Can you work these out from the drawing? Everything is in mm from the part's minimum corner. A direction names the side the tool comes from. Round coordinates to 2 decimals unless told otherwise and drop trailing zeros. Loops run counter-clockwise (first coordinate to the right, second up) from the corner with the lowest first, then second, coordinate; pieces in that order, holes last. Notation, with made-up numbers: (56.5, 6) - (108.5, 6) arc R5 ccw to (108.5, 10) - close; hole circle Ø11 at (55.25, -19). An arc over 180 degrees is marked (long way). Answer as a JSON object with one key per item and string values. Group by question number.
1) I want a section at B-B, the plane x = 30.5. Please give me the cut outline in (y, z) (3 decimals), then the cut area to 3 significant figures.
2) I want a section at C-C, the plane y = 28. Please give me the cut outline in (x, z) (3 decimals).
3) If I drill on line 1 along Z through (x, y) = (15.5, 2) (3 decimals); line 2 along X through (y, z) = (18, 12.5); line 3 along Z through (x, y) = (21, 7.5) (3 decimals), over which ranges is the centre line in solid material (lowest first)? Write a range as [from, to].
4) I want a section at D-D, the plane z = 10. Please give me the cut outline in (x, y) (1 decimal), then the cut area to 3 significant figures.
5) If we mould it in two halves opening along Z, with no side actions, what happens to the marked faces 4, 5, 6 and 7? For each: pulls with the +Z half, pulls with the -Z half, needs draft (parallel to the pull), parting line crosses it, or undercut.
6) Which directions (+Z, -Z, +X, -X, +Y, -Y) give clear straight access to the entire face, cutting with the end or side of a thin tool? Please do the marked faces 1, 2 and 3.
7) Will these pins go through, and if not, where does the flat tip stop? P1, Ø16, axis at x = 8, y = 23, coming from the -Z side; P2, Ø1, axis at y = 12.5, z = 4, coming from the -X side; P3, Ø4, axis at y = 20, z = 18.5, coming from the +X side.
8) I want a section at A-A, the plane x = 12. Please give me the cut outline in (y, z) (3 decimals).
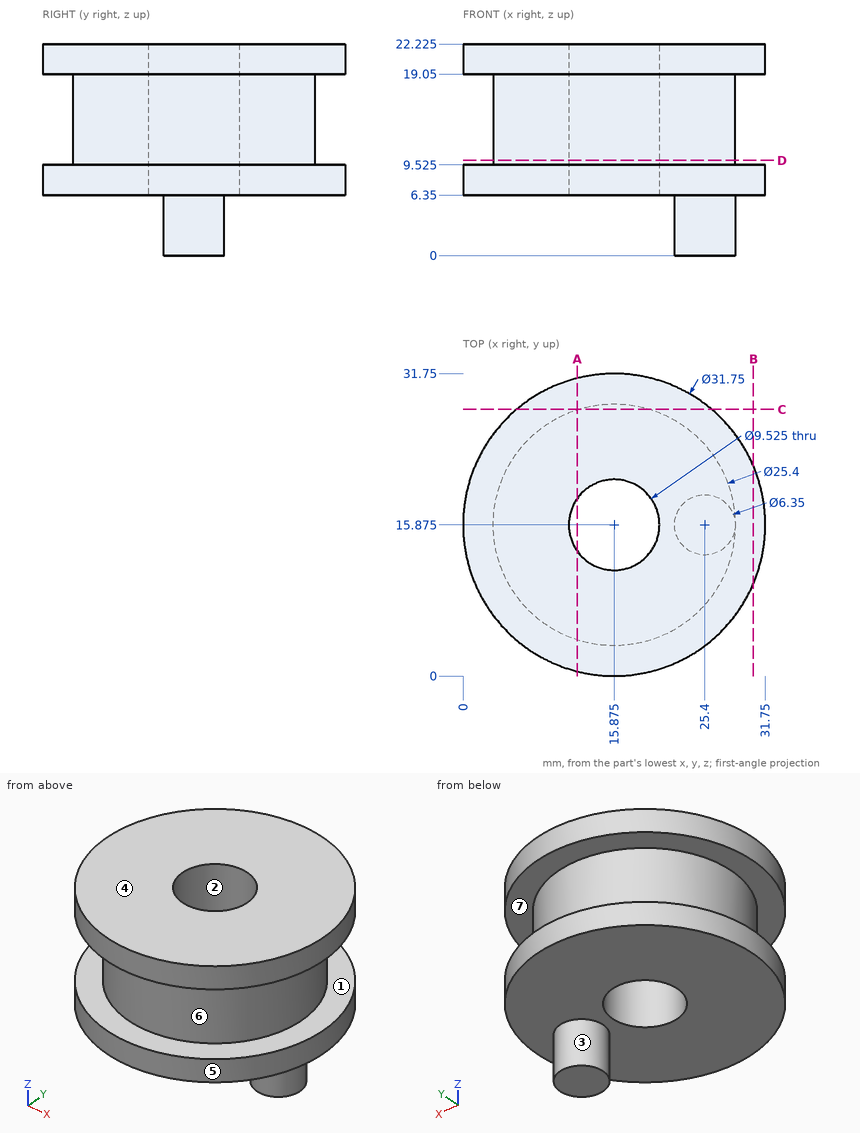
Outcome:
{
 "1": {"outline": "(9.7, 6.35) - (22.05, 6.35) - (22.05, 9.525) - (9.7, 9.525) - close; (9.7, 19.05) - (22.05, 19.05) - (22.05, 22.225) - (9.7, 22.225) - close", "area": "78.4 mm^2"},
 "2": {"outline": "(5.628, 6.35) - (26.122, 6.35) - (26.122, 9.525) - (19.653, 9.525) - (19.653, 19.05) - (26.122, 19.05) - (26.122, 22.225) - (5.628, 22.225) - (5.628, 19.05) - (12.097, 19.05) - (12.097, 9.525) - (5.628, 9.525) - close"},
 "3": {"line 1": "[6.35, 9.525], [19.05, 22.225]", "line 2": "[3.35, 11.61], [20.14, 28.4]", "line 3": "[6.35, 22.225]"},
 "4": {"outline": "circle Ø25.4 at (15.9, 15.9); hole circle Ø9.5 at (15.9, 15.9)", "area": "435 mm^2"},
 "5": {"face 4": "pulls with the +Z half", "face 5": "needs draft", "face 6": "undercut", "face 7": "undercut"},
 "6": {"face 1": "none", "face 2": "+Z, -Z", "face 3": "-Z"},
 "7": {"P1": "z = 6.35", "P2": "x = 24.05", "P3": "x = 31.6"},
 "8": {"outline": "(0.48, 6.35) - (13.106, 6.35) - (13.106, 22.225) - (0.48, 22.225) - (0.48, 19.05) - (3.781, 19.05) - (3.781, 9.525) - (0.48, 9.525) - close; (18.644, 6.35) - (31.27, 6.35) - (31.27, 9.525) - (27.969, 9.525) - (27.969, 19.05) - (31.27, 19.05) - (31.27, 22.225) - (18.644, 22.225) - close"}
}
